from build123d import *

# Parameters (mm, degrees)
F0_R       = 10
F1_DEPTH   = 4
F2_R       = 4.85
F3_DEPTH   = 3.5
F4_R       = 6.95
F4_R_2     = 6
F5_DEPTH   = 0.5
F6_R       = 10
F6_R_2     = 6.95
F7_DEPTH   = 3
F8_SIZE    = 0.25
F9_SIZE2   = 0.99999
F9_SIZE    = 0.49999
F9_2_SIZE2 = 1
F9_2_SIZE  = 0.5


# Not quite as in the source:
# - a fillet or chamfer is up to 0.001 mm smaller than in the source, because OpenCascade refuses the exact size


with BuildPart() as f1:
    # F0 (on Right) → F1 (new body)
    with BuildSketch(Plane.YZ):
        Circle(F0_R)
    extrude(amount=F1_DEPTH)

    # F2 (on face) → F3 (join)
    with BuildSketch(Plane(origin=(0, 0, 0), x_dir=(0, -1, 0), z_dir=(-1, 0, 0))):
        Circle(F2_R)
    extrude(amount=F3_DEPTH)

    # F4 (on face) → F5 (join)
    with BuildSketch(Plane(origin=(0, 0, 0), x_dir=(0, -1, 0), z_dir=(-1, 0, 0))):
        Circle(F4_R)
        Circle(F4_R_2, mode=Mode.SUBTRACT)
    extrude(amount=F5_DEPTH)

    # F6 (on face) → F7 (cut)
    with BuildSketch(Plane(origin=(0, 0, 0), x_dir=(0, -1, 0), z_dir=(-1, 0, 0))):
        Circle(F6_R)
        Circle(F6_R_2, mode=Mode.SUBTRACT)
    extrude(amount=-F7_DEPTH, mode=Mode.SUBTRACT)

    # F8
    f8_edges = [f1.edges().sort_by_distance(p)[0] for p in [
        (-0.5, 6.95, 0),
        (-0.5, 6, 0),
    ]]
    chamfer(f8_edges, length=F8_SIZE)

    # F9 (size 0.5 and 1 in the source; OpenCascade refuses exactly that, so slightly less here)
    f9_edges = [f1.edges().sort_by_distance(p)[0] for p in [
        (4, -10, 0),
    ]]
    f9_side = f1.faces().sort_by_distance((4, 0, 0))[0]
    chamfer(f9_edges, length=F9_SIZE, length2=F9_SIZE2, reference=f9_side)

    # F9#2
    f9_2_edges = [f1.edges().sort_by_distance(p)[0] for p in [
        (-3.5, 4.85, 0),
    ]]
    f9_2_side = f1.faces().sort_by_distance((-3.5, 0, 0))[0]
    chamfer(f9_2_edges, length=F9_2_SIZE, length2=F9_2_SIZE2, reference=f9_2_side)


solid = f1.part
Part model, mm, in its own coordinate system. A direction names the side the tool comes from. Round coordinates to 2 decimals unless told otherwise and drop trailing zeros. Loops run counter-clockwise (first coordinate to the right, second up) from the corner with the lowest first, then second, coordinate; pieces in that order, holes last. Notation, with made-up numbers: (21.25, -28.75) - (59.25, -28.75) arc R14 cw to (59.25, -1.75) - close; hole circle Ø6 at (65, -8). An arc over 180 degrees is marked (long way). Answer as a JSON object with one key per item and string values.
Item 1: Pin check, flat tips, straight feed: pin 1 (3 mm diameter, centred on x = -1, y = -2.5, fed in from +Z); pin 2 (3 mm diameter, centred on y = 3, z = -7.5, fed in from -X). Stop position of each tip, or through.
Output:
{"pin 1": "z = 6.85", "pin 2": "x = -0.5"}
Item 2: Band-saw the part on C-C on x = 3.5. List the corners of the cut face in (y, z).
Output:
{"outline": "circle Ø19.5 at (0, 0)"}
Item 3: Wall check: L1, parallel to Z at x = -0.2, y = 0; L2, parallel to X at y = 7.75, z = -4.5; L3, parallel to X at y = -1.5, z = 5.75. Give the ranges that are in metal, low to high.
Output:
{"L1": "-6.95 to -6, -4.85 to 4.85, 6 to 6.95", "L2": "3 to 4", "L3": "0 to 4"}
Item 4: Pull direction Y, two halves, no side cores. Call faces 1 (the face through (-3.5, 0, 0)), 2 (the face through (1.352, 1.507, -6.785)), 3 (the face through (0, 5, 0)): pulls with the +Y half, pulls with the -Y half, needs draft (parallel to the pull), parting line crosses it, or undercut.
Output:
{"face 1": "needs draft", "face 2": "parting line crosses it", "face 3": "undercut"}
Item 5: Band-saw the part on D-D on x = -1.5. List the corners of the cut face in (y, z).
Output:
{"outline": "circle Ø9.7 at (0, 0)"}
Item 6: Tool access for faces 4 (the face through (4, 0, 0)), 5 (the face through (3, -2, 7)): list every direction of +Z, -Z, +X, -X, +Y, -Y with a clear straight run to the whole face (end or side of a thin tool).
Output:
{"face 4": "+Z, -Z, +X, +Y, -Y", "face 5": "-X"}
